Model file for the job. Use its own axes, mm. Face numbers are marked on the shaded views. Give positions to 0.01 mm unless a question says otherwise; leave off trailing zeros. Loops run counter-clockwise (first coordinate to the right, second up) from the corner with the lowest first, then second, coordinate; pieces in that order, holes last. Notation, with made-up numbers: M 37,80 L 63,80 A16 ccw 63,92 Z; hole C -19,41 d4. An arc over 180 degrees is marked long. Use CSV: the item, a comma, the result in double quotes. Start each with the question number.
(1) Slice it at C-C on y = 10. List the corners of the cut face in (x, z).
(2) Slice it at A-A on z = 0.3. List the corners of the cut face in (x, y).
(3) Slice it at B-B on x = -47.5. List the corners of the cut face in (y, z).
(4) Wall check: line 1 along Y through (x, z) = (-8, 0.1); line 2 along Z through (x, y) = (-33.5, 12); line 3 along X through (y, z) = (17, 0.9). Give the ranges that are in metal, low to high. Write a range as from..to.
(5) Flat gauge pin, fed straight in: P1, Ø1.5, axis at x = -63.5, y = -18, coming from the +Z side. Where does the tip first touch, or does it go through?
(6) Two-plate mould, pull along Y, no slides. Class the marked faces 1 and 2: pulls with the +Y half, pulls with the -Y half, needs draft (parallel to the pull), parting line crosses it, or undercut.
```python
from build123d import *

# Parameters (mm, degrees)
F0_W     = 100
F0_H     = 38
F1_DEPTH = 0.5
F2_W     = 100
F2_H     = 3
F3_DEPTH = 0.8
F4_R     = 0.75
F5_DEPTH = 0.5
F6_R     = 0.75
F7_DEPTH = 0.5


# Not quite as in the source:
# - a feature names something its author has since deleted; it is built from what else it names


with BuildPart() as f1:
    # F0 (on Top) → F1 (new body)
    with BuildSketch(Plane.XY):
        with Locations((-50, 0)):
            Rectangle(F0_W, F0_H)
    extrude(amount=-F1_DEPTH)

    # F2 (on face) → F3 (join)
    with BuildSketch(Plane.XY):
        with Locations((-50, 17.5)):
            Rectangle(F2_W, F2_H)
        with Locations((-50, -17.5)):
            Rectangle(F2_W, F2_H)
    extrude(amount=F3_DEPTH)

    # F4 (on face) → F5 (join)
    with BuildSketch(Plane.XY.offset(0.8)):
        with Locations((-95, 17.5)):
            Circle(F4_R)
        with Locations((-72.5, 17.5)):
            Circle(F4_R)
        with Locations((-50, 17.5)):
            Circle(F4_R)
        with Locations((-27.5, 17.5)):
            Circle(F4_R)
        with Locations((-5, 17.5)):
            Circle(F4_R)
    extrude(amount=F5_DEPTH)

    # F6 (on face) → F7 (join)
    with BuildSketch(Plane.XY.offset(0.8)):
        with Locations((-95, -17.5)):
            Circle(F6_R)
        with Locations((-72.5, -17.5)):
            Circle(F6_R)
        with Locations((-50, -17.5)):
            Circle(F6_R)
        with Locations((-27.5, -17.5)):
            Circle(F6_R)
        with Locations((-5, -17.5)):
            Circle(F6_R)
    extrude(amount=F7_DEPTH)


solid = f1.part
```
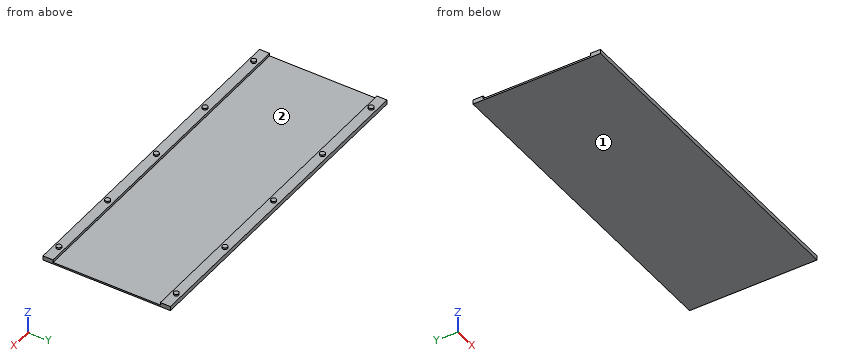
Reply:
1,outline,"M -100,-0.5 L 0,-0.5 L 0,0 L -100,0 Z"
2,outline,"M -100,-19 L 0,-19 L 0,-16 L -100,-16 Z; M -100,16 L 0,16 L 0,19 L -100,19 Z"
3,outline,"M -19,-0.5 L 19,-0.5 L 19,0.8 L 16,0.8 L 16,0 L -16,0 L -16,0.8 L -19,0.8 Z"
4,line 1,"y = -19..-16, 16..19"
4,line 2,"z = -0.5..0"
4,line 3,"x = -95.56..-94.44, -73.06..-71.94, -50.56..-49.44, -28.06..-26.94, -5.56..-4.44"
5,P1,"stops at z = 0.8"
6,face 1,"needs draft"
6,face 2,"undercut"
